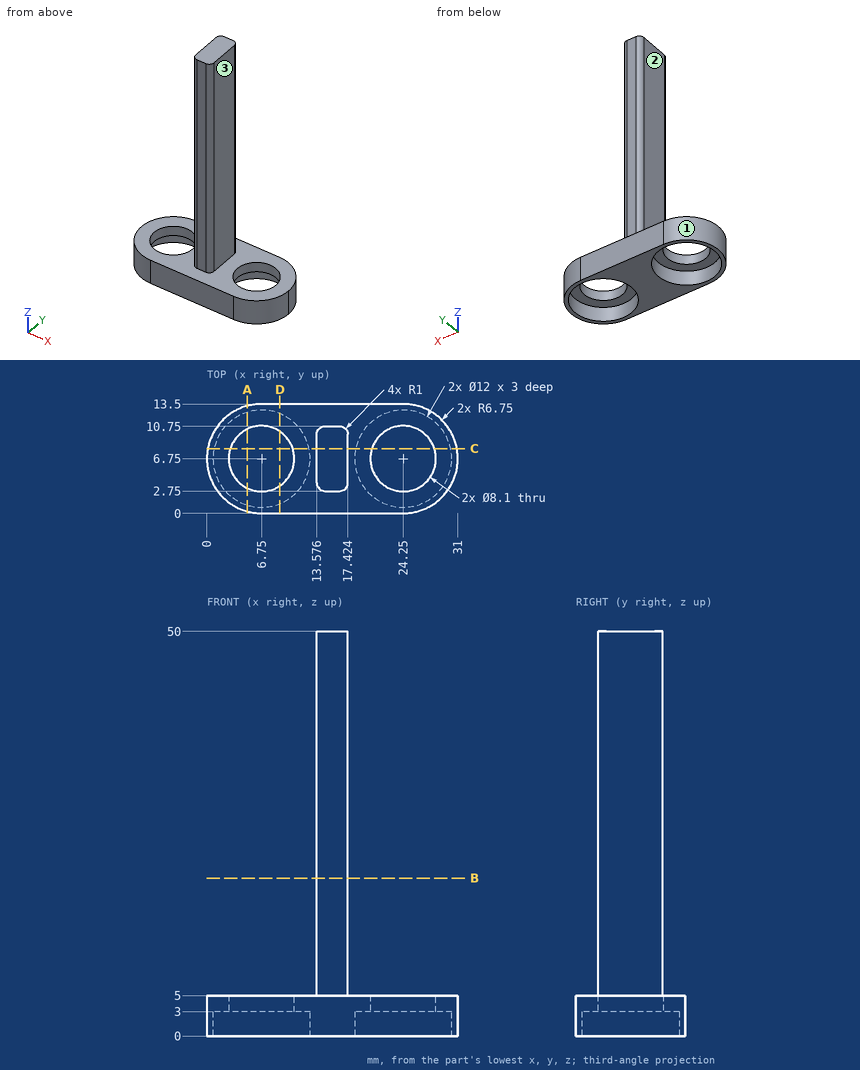
Geometry: see drawing. Coordinates: mm, zero at the bounding-box minimum. A direction names the side the tool comes from. Coordinates: 2 decimals unless noted, no trailing zeros. Order: outer loops, then holes, each group sorted by start corner. A loop starts at its lowest first (then second) coordinate and runs counter-clockwise, first axis right, second up. Notation, with made-up numbers: M 52.25,57.5 L 76.25,57.5 A14 ccw 76.25,81.5 Z; hole C 76.25,-26 d8. An arc over 180 degrees is marked long. Write item = value, one per line. Start each with the question number.
(1) Section B-B on z = 19.5. Output: boundary loops of the cut face in (x, y).
(2) Reachability of the marked faces 1, 2 and 3 from +Z, -Z, +X, -X, +Y, -Y: full face, straight path, thin tool, end or side. Return the list, or none.
(3) Section D-D on x = 9. Output: boundary loops of the cut face in (y, z), and give its area (3 significant figures).
(4) Section C-C on y = 8. Output: boundary loops of the cut face in (x, z), and give its area (3 significant figures).
(5) First-contact query: P1, Ø1.8, axis at y = 7, z = 24, coming from the +X side; P2, Ø5, axis at x = 4.5, y = 9, coming from the +Z side; P3, Ø0.6, axis at x = 15.5, z = 33, coming from the -Y side. Flat tips, straight axial feed; report the tip coordinate or a pass-through.
(6) Line query: line 1 along Y through (x, z) = (24.25, 3.55); line 2 along Z through (x, y) = (17.5, 11); line 3 along X through (y, z) = (5.25, 15.5). Output: solid intervals per line, ascending. Write a range as [from, to].
(7) Section A-A on x = 5. Output: boundary loops of the cut face in (y, z), and give its area (3 significant figures).
Result set:
q1.outline = M 13.58,3.75 A1 ccw 14.58,2.75 L 16.42,2.75 A1 ccw 17.42,3.75 L 17.42,9.75 A1 ccw 16.42,10.75 L 14.58,10.75 A1 ccw 13.58,9.75 Z
q2.face_1 = +Z, -Z, -X
q2.face_2 = +Z, -X, +Y, -Y
q2.face_3 = +Z, +X, +Y, -Y
q3.outline = M 0,0 L 1.19,0 L 1.19,3 L 3.38,3 L 3.38,5 L 0,5 Z; M 10.12,3 L 12.31,3 L 12.31,0 L 13.5,0 L 13.5,5 L 10.12,5 Z
q3.area = 20.7 mm²
q4.outline = M 0.12,0 L 0.88,0 L 0.88,3 L 2.9,3 L 2.9,5 L 0.12,5 Z; M 10.6,3 L 12.62,3 L 12.62,0 L 18.38,0 L 18.38,3 L 20.4,3 L 20.4,5 L 17.42,5 L 17.42,50 L 13.58,50 L 13.58,5 L 10.6,5 Z; M 28.1,3 L 30.12,3 L 30.12,0 L 30.88,0 L 30.88,5 L 28.1,5 Z
q4.area = 226 mm²
q5.P1 = 17.42
q5.P2 = 5
q5.P3 = 2.75
q6.line_1 = [0, 2.7], [10.8, 13.5]
q6.line_2 = [0, 5]
q6.line_3 = [13.58, 17.42]
q7.outline = M 0.23,0 L 1.01,0 L 1.01,3 L 3.1,3 L 3.1,5 L 0.23,5 Z; M 10.4,3 L 12.49,3 L 12.49,0 L 13.27,0 L 13.27,5 L 10.4,5 Z
q7.area = 16.1 mm²
